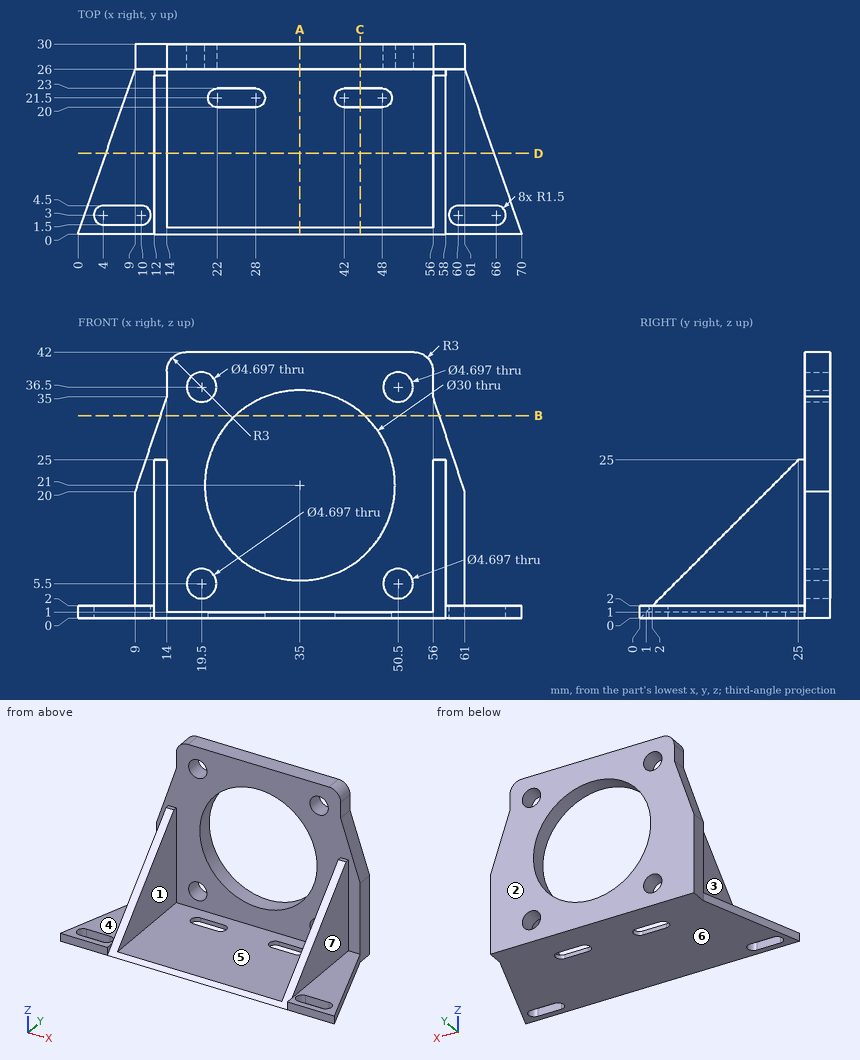
The drawing under review shows one solid part. Ordinate dimensions are in mm from its lowest x, y, z. A direction names the side the tool comes from. Coordinates: 2 decimals unless noted, no trailing zeros. Order: outer loops, then holes, each group sorted by start corner. A loop starts at its lowest first (then second) coordinate and runs counter-clockwise, first axis right, second up. Notation, with made-up numbers: (-39.75, -2) -> (-19.75, -2) arc R15 cw to (-19.75, 5) -> close; hole circle Ø2 at (68, 13.5). An arc over 180 degrees is marked (long way). Answer in a Markdown table with one row per item.
(1) Insertion check: pin 1 (5 mm diameter, centred on y = 23, z = 22, fed in from -X); pin 2 (1.5 mm diameter, centred on x = 55, z = 13.5, fed in from -Y); pin 3 (1.2 mm diameter, centred on y = 28, z = 36, fed in from -X). Each pin has a flat end and moves straight along its axis. Give the tip position at first contact, or say it passes through.
Answers:
| item | result |
|---|---|
| pin 1 | x = 12 |
| pin 2 | y = 26 |
| pin 3 | x = 14 |
(2) Machinability: for the marked faces 4, 5, 6 and 7, which of the approach directions +Z, -Z, +X, -X, +Y, -Y give a long, thin tool a straight path to every point of the face, cutting with its end or side? Answer none if there is none.
Answers:
| item | result |
|---|---|
| face 4 | +Z, -X, -Y |
| face 5 | +Z, -Y |
| face 6 | -Z, +X, -X, +Y, -Y |
| face 7 | +Z, +X, -Y |
(3) The part is to be moulded in two halves that separate along X. For the marked faces 1, 2 and 3, say which applies: +X half, -X half, draft (parallel to the pull), parting line (faces both ways), or undercut.
Answers:
| item | result |
|---|---|
| face 1 | undercut |
| face 2 | draft |
| face 3 | -X half |
(4) Consider section A-A (x = 35). Write out the cut boundary in (y, z).
Answers:
| item | result |
|---|---|
| outline | (0, 0) -> (30, 0) -> (30, 6) -> (26, 6) -> (26, 1) -> (1, 1) -> close; (26, 36) -> (30, 36) -> (30, 42) -> (26, 42) -> close |
(5) Wall thickness on line 1 along Z through (x, y) = (50.5, 27.85); line 2 along Z through (x, y) = (35, 27.15); line 3 along X through (y, z) = (20.5, 6): over which ranges is each line inside the solid? List them lowest first.
Answers:
| item | result |
|---|---|
| line 1 | 0 to 3.15, 7.85 to 34.15, 38.85 to 42 |
| line 2 | 0 to 6, 36 to 42 |
| line 3 | 12 to 14, 56 to 58 |
(6) Consider section C-C (x = 44.5). Write out the cut boundary in (y, z).
Answers:
| item | result |
|---|---|
| outline | (0, 0) -> (20, 0) -> (20, 1) -> (1, 1) -> close; (23, 0) -> (30, 0) -> (30, 9.39) -> (26, 9.39) -> (26, 1) -> (23, 1) -> close; (26, 32.61) -> (30, 32.61) -> (30, 42) -> (26, 42) -> close |
(7) Consider section B-B (z = 32). Write out the cut boundary in (x, y).
Answers:
| item | result |
|---|---|
| outline | (13, 26) -> (24.8, 26) -> (24.8, 30) -> (13, 30) -> close; (45.2, 26) -> (57, 26) -> (57, 30) -> (45.2, 30) -> close |
(8) Consider section D-D (y = 12.75). Write out the cut boundary in (x, z).
Answers:
| item | result |
|---|---|
| outline | (4.41, 0) -> (65.59, 0) -> (65.59, 2) -> (58, 2) -> (58, 12.75) -> (56, 12.75) -> (56, 1) -> (14, 1) -> (14, 12.75) -> (12, 12.75) -> (12, 2) -> (4.41, 2) -> close |
